from build123d import *

# Parameters (mm, degrees)
SKETCH1_W           = 60
SKETCH1_H           = 57
SKETCH1_W_2         = 14
SKETCH1_H_2         = 14
SKETCH1_W_3         = 37
SKETCH1_H_3         = 12
SKETCH1_W_4         = 6
SKETCH1_H_4         = 6
BOSS_EXTRUDE1_DEPTH = 1.5


with BuildPart() as part:
    # Sketch1 → Boss-Extrude1 (new body)
    with BuildSketch(Plane.XY):
        with Locations((0.299968287, -12.658536585)):
            Rectangle(SKETCH1_W, SKETCH1_H)
        with Locations((-18.700031713, -30.158536585)):
            Rectangle(SKETCH1_W_2, SKETCH1_H_2, mode=Mode.SUBTRACT)
        with Locations((0.299968287, -30.158536585)):
            Rectangle(SKETCH1_W_2, SKETCH1_H_2, mode=Mode.SUBTRACT)
        with Locations((19.299968287, -30.158536585)):
            Rectangle(SKETCH1_W_2, SKETCH1_H_2, mode=Mode.SUBTRACT)
        with Locations((0.085273165, -11.158536585)):
            Rectangle(SKETCH1_W_2, SKETCH1_H_2, mode=Mode.SUBTRACT)
        with Locations((0.299968287, 5.841463415)):
            Rectangle(SKETCH1_W_3, SKETCH1_H_3, mode=Mode.SUBTRACT)
        with Locations((-18.700031713, -11.158536585)):
            Rectangle(SKETCH1_W_4, SKETCH1_H_4, mode=Mode.SUBTRACT)
        with Locations((19.299968287, -11.158536585)):
            Rectangle(SKETCH1_W_4, SKETCH1_H_4, mode=Mode.SUBTRACT)
    extrude(amount=BOSS_EXTRUDE1_DEPTH)


solid = part.part
Model file for the job. Use its own axes, mm. A direction names the side the tool comes from. Round coordinates to 2 decimals unless told otherwise and drop trailing zeros. Loops run counter-clockwise (first coordinate to the right, second up) from the corner with the lowest first, then second, coordinate; pieces in that order, holes last.
1. Band-saw the part on C-C, the plane y = 9.5. List the corners of the cut face in (x, z), and give its area (3 significant figures).
Check values:
outline: (-29.7, 0) - (-18.2, 0) - (-18.2, 1.5) - (-29.7, 1.5) - close; (18.8, 0) - (30.3, 0) - (30.3, 1.5) - (18.8, 1.5) - close
area: 34.5 mm2
2. Tool access for faces 1 (the flat face through (0, -41.159, 1)), 2 (the flat face through (19, -37.159, 1)): list every direction of +Z, -Z, +X, -X, +Y, -Y with a clear straight run to the whole face (end or side of a thin tool).
Check values:
face 1: +Z, -Z, +X, -X, -Y
face 2: +Z, -Z
3. Band-saw the part on B-B, the plane z = 0.45. Count the separate pieces of the cut face and the enclosed holes in it, and give its area (3 significant figures).
Check values:
separate pieces: 1
enclosed holes: 7
area: 2,120 mm2
4. Band-saw the part on A-A, the plane x = -24. List the corners of the cut face in (y, z), and give its area (3 significant figures).
Check values:
outline: (-41.16, 0) - (-37.16, 0) - (-37.16, 1.5) - (-41.16, 1.5) - close; (-23.16, 0) - (15.84, 0) - (15.84, 1.5) - (-23.16, 1.5) - close
area: 64.5 mm2
5. Mould opens along Y. For faces 3 (the flat face through (0, 15.841, 1)), 4 (the flat face through (26.3, -30, 1)), 5 (the flat face through (30.3, -13, 1)) say: +Y half, -Y half, draft (parallel to the pull), parting line (faces both ways), or undercut.
Check values:
face 3: +Y half
face 4: undercut
face 5: draft
6. Wall check: probe 1 along Y at (x, z) = (1.5, 0.7); probe 2 along Y at (x, z) = (14, 0.9); probe 3 along X at (y, z) = (-33, 0.25). Give the ranges that are in metal, low to high.
Check values:
probe 1: y = -41.16 to -37.16, -23.16 to -18.16, -4.16 to -0.16, 11.84 to 15.84
probe 2: y = -41.16 to -37.16, -23.16 to -0.16, 11.84 to 15.84
probe 3: x = -29.7 to -25.7, -11.7 to -6.7, 7.3 to 12.3, 26.3 to 30.3
7. Band-saw the part on D-D, the plane x = 5.5. List the corners of the cut face in (y, z).
Check values:
outline: (-41.16, 0) - (-37.16, 0) - (-37.16, 1.5) - (-41.16, 1.5) - close; (-23.16, 0) - (-18.16, 0) - (-18.16, 1.5) - (-23.16, 1.5) - close; (-4.16, 0) - (-0.16, 0) - (-0.16, 1.5) - (-4.16, 1.5) - close; (11.84, 0) - (15.84, 0) - (15.84, 1.5) - (11.84, 1.5) - close
